Geometry check sheet. Reference: the model listing, model coordinates, mm. Face numbers are marked on the shaded views. A direction names the side the tool comes from. Round coordinates to 2 decimals unless told otherwise and drop trailing zeros. Order: outer loops, then holes, each group sorted by start corner. A loop starts at its lowest first (then second) coordinate and runs counter-clockwise, first axis right, second up. Notation, with made-up numbers: (57, -19.5) - (64, -19.5) arc R33 cw to (64, 19.5) - close; hole circle Ø9 at (10.5, 27). An arc over 180 degrees is marked (long way). Return JSON: item names as keys, results as strings. Group by question number.
Q1. Tool access check on the marked faces 4, 5, 6 and 7. Record the directions out of +Z, -Z, +X, -X, +Y, -Y that give a thin tool (end or side, any length) a straight path to the whole face; none if there is none.
Q2. Gauge pin test, flat ends, axial feed: pin 1 Ø6 at (x, z) = (3.5, 12.5) entering from -Y; pin 2 Ø3.5 at (x, z) = (-11.68, 6.74) entering from +Y; pin 3 Ø2 at (y, z) = (5, 13) entering from -X; pin 4 Ø3 at (x, y) = (-3, 4.5) entering from +Z. Record the tip position at first contact, or that the pin passes through.
Q3. Sectioned sample at A-A, the plane z = -6. Record the cut outline in (x, y).
Q4. Sectioned sample at D-D, the plane x = -10.5. Record the cut outline in (y, z).
Q5. Sectioned sample at B-B, the plane x = -2.75. Record the cut outline in (y, z), then the cut area to 3 significant figures.
Q6. Draft check along Z on the marked faces 1, 2 and 3. Enter one of: pulls with the +Z half, pulls with the -Z half, needs draft (parallel to the pull), parting line crosses it, or undercut.
Q7. Sectioned sample at C-C, the plane y = 4. Record the cut outline in (x, z).
Q8. Material ranges on line 1 along Z through (x, y) = (0, 4.7); line 2 along Z through (x, y) = (-13.5, 0.5); line 3 along Z through (x, y) = (-11, 2.25), recorded low to high.
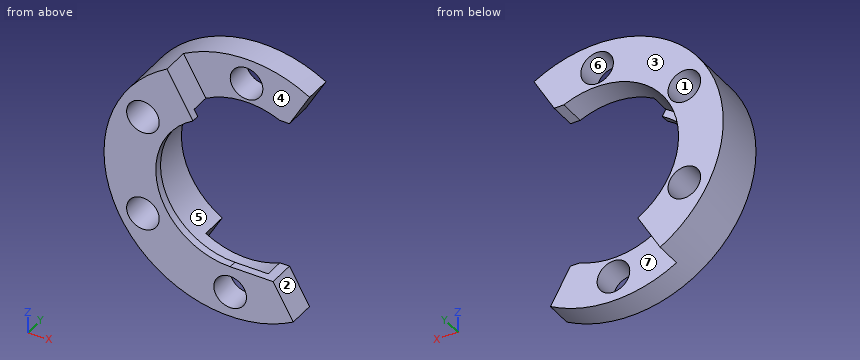
```python
from build123d import *

# Parameters (mm, degrees)
SKETCH1_R         = 16.891
EXTRUDE1_DEPTH    = 7.239
SKETCH2_R         = 10.9093
EXTRUDE2_DEPTH    = 25.960266084
SKETCH3_R         = 10.9093
SKETCH3_R_2       = 9.9568
EXTRUDE3_DEPTH    = 1.0414
SKETCH4_R         = 2.1844
EXTRUDE4_DEPTH    = 25.960266084
CIRPATTERN1_COUNT = 6
SKETCH5_W         = 23.383447214
SKETCH5_H         = 19.9136
EXTRUDE6_DEPTH    = 25.960266084
EXTRUDE7_DEPTH    = 25.960266084
EXTRUDE8_DEPTH    = 3.6195
EXTRUDE9_DEPTH    = 3.6195


with BuildPart() as part:
    # Sketch1 → Extrude1 (new body)
    with BuildSketch(Plane(origin=(0, 0, 0), x_dir=(1, 0, 0), z_dir=(0, 1, 0))):
        with Locations(Location((0, 0, 0), (0, 0, 270))):
            Circle(SKETCH1_R)
    extrude(amount=EXTRUDE1_DEPTH)

    # Sketch2 → Extrude2 (cut, through all)
    with BuildSketch(Plane.XZ):
        with Locations(Location((0, 0, 0), (0, 0, 270))):
            Circle(SKETCH2_R)
    extrude(amount=-EXTRUDE2_DEPTH, mode=Mode.SUBTRACT)

    # Sketch3 → Extrude3 (add)
    with BuildSketch(Plane.XZ):
        with Locations(Location((0, 0, 0), (0, 0, 270))):
            Circle(SKETCH3_R)
        with Locations(Location((0, 0, 0), (0, 0, 270))):
            Circle(SKETCH3_R_2, mode=Mode.SUBTRACT)
    extrude(amount=-EXTRUDE3_DEPTH)

    # Sketch4 → Extrude4 (cut, through all)
    with BuildSketch(Plane(origin=(0, 7.239, 0), x_dir=(1, 0, 0), z_dir=(0, 1, 0))):
        with Locations(Location((0, 13.4874, 0), (0, 0, 270))):
            Circle(SKETCH4_R)
    extrude4 = extrude(amount=-EXTRUDE4_DEPTH, mode=Mode.SUBTRACT)

    # CirPattern1: Extrude4 ×6 about axis
    cirpattern1_axis = Axis((0, 0, 0), (0, 1, 0))
    for i in range(1, CIRPATTERN1_COUNT):
        add(extrude4.rotate(cirpattern1_axis, i * 360 / CIRPATTERN1_COUNT), mode=Mode.SUBTRACT)

    # Sketch5 → Extrude6 (cut, through all)
    with BuildSketch(Plane(origin=(0, 7.239, 0), x_dir=(1, 0, 0), z_dir=(0, 1, 0))):
        with Locations((11.691723607, 0)):
            Rectangle(SKETCH5_W, SKETCH5_H)
    extrude(amount=-EXTRUDE6_DEPTH, mode=Mode.SUBTRACT)

    # Sketch8 → Extrude7 (cut, through all)
    with BuildSketch(Plane(origin=(0, 7.239, 0), x_dir=(1, 0, 0), z_dir=(0, 1, 0))):
        Polygon((0, 0), (17.025211733, 0), (17.025211733, 29.488531731), align=None)
    extrude7 = extrude(amount=-EXTRUDE7_DEPTH, mode=Mode.SUBTRACT)

    # Mirror1: Extrude7 across plane
    add(extrude7.mirror(Plane.XY), mode=Mode.SUBTRACT)

    # Sketch9 → Extrude8 (cut)
    with BuildSketch(Plane(origin=(0, 7.239, 0), x_dir=(1, 0, 0), z_dir=(0, 1, 0))):
        Polygon((0, 0), (-11.081515353, 19.193747616), (11.081515353, 19.193747616), align=None)
    extrude(amount=-EXTRUDE8_DEPTH, mode=Mode.SUBTRACT)

    # Sketch10 → Extrude9 (cut)
    with BuildSketch(Plane.XZ):
        Polygon((0, 0), (-13.504747016, 23.390907976), (14.410908918, 24.960426429), align=None)
    extrude(amount=-EXTRUDE9_DEPTH, mode=Mode.SUBTRACT)


solid = part.part
```
Reply:
{
 "1": {"face 4": "+Z, +X, -Y", "face 5": "+Y", "face 6": "+Y, -Y", "face 7": "-Z, +X, +Y"},
 "2": {"pin 1": "y = 3.62", "pin 2": "through", "pin 3": "x = -11.89", "pin 4": "z = 16.82"},
 "3": {"outline": "(-15.79, 0) - (-13.73, 0) - (-13.73, 7.24) - (-15.79, 7.24) - close; (-9.63, 0) - (-7.95, 0) - (-7.95, 1.04) - (-9.11, 1.04) - (-9.11, 7.24) - (-9.63, 7.24) - close"},
 "4": {"outline": "(0, -13.23) - (7.24, -13.23) - (7.24, -8.58) - (0, -8.58) - close; (0, -4.91) - (7.24, -4.91) - (7.24, -2.96) - (1.04, -2.96) - (1.04, 2.96) - (7.24, 2.96) - (7.24, 4.91) - (0, 4.91) - close; (0, 8.58) - (7.24, 8.58) - (7.24, 13.23) - (0, 13.23) - close"},
 "5": {"outline": "(0, -16.67) - (3.62, -16.67) - (3.62, -10.56) - (1.04, -10.56) - (1.04, -9.57) - (0, -9.57) - close; (3.62, 10.56) - (7.24, 10.56) - (7.24, 16.67) - (3.62, 16.67) - close", "area": "45.2 mm^2"},
 "6": {"face 1": "undercut", "face 2": "pulls with the +Z half", "face 3": "needs draft"},
 "7": {"outline": "(-8.45, -14.63) - (-5.45, -9.45) arc R10.91 cw to (4.46, 9.96) - (5.75, 9.96) - (8.45, 14.63) arc R16.89 ccw to start; hole circle Ø4.37 at (-11.68, -6.74); hole circle Ø4.37 at (-11.68, 6.74); hole circle Ø4.37 at (0, 13.49)"},
 "8": {"line 1": "10.91 to 11.3, 15.67 to 16.89", "line 2": "-10.15 to -7.95, -5.54 to 5.54, 7.95 to 10.15", "line 3": "-12.82 to -8.82, -4.67 to 4.67, 8.82 to 12.82"}
}
